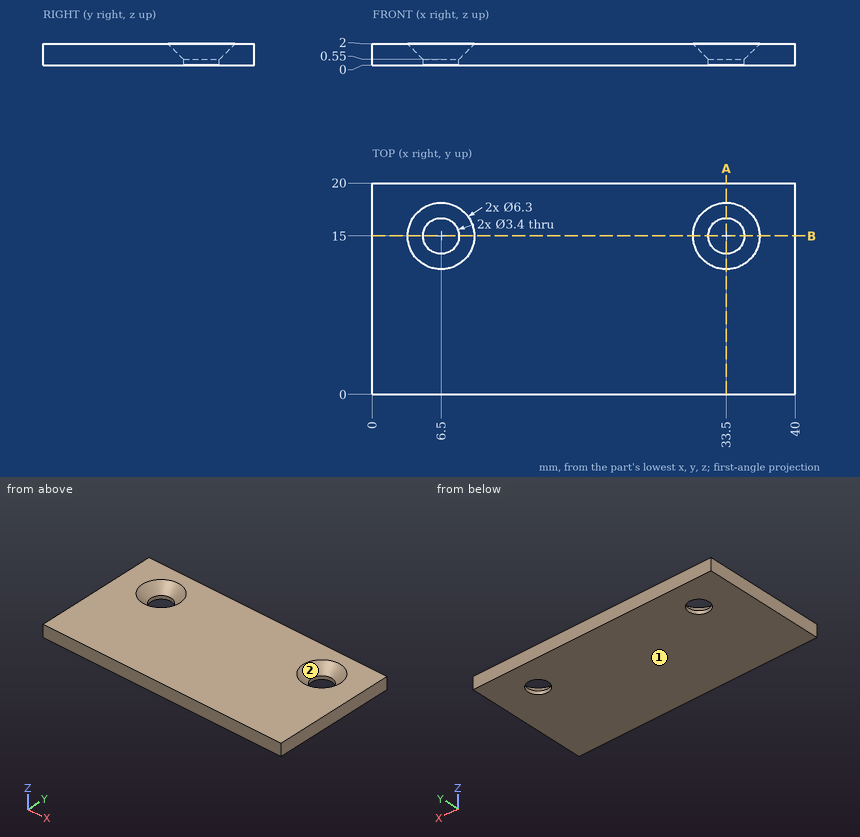
The drawing under review shows one solid part. Ordinate dimensions are in mm from its lowest x, y, z. Coordinates: 2 decimals unless noted, no trailing zeros. Order: outer loops, then holes, each group sorted by start corner. A loop starts at its lowest first (then second) coordinate and runs counter-clockwise, first axis right, second up. Notation, with made-up numbers: M 3,56.5 L 15,56.5 A21 ccw 15,93.5 Z; hole C -38,34 d6. An arc over 180 degrees is marked long. Use a Markdown table: item, result.
(1) Add section A-A (x = 33.5). Give the boundary of the cut face in (y, z).
Worked answers:
| item | result |
|---|---|
| outline | M 0,0 L 13.3,0 L 13.3,0.55 L 11.85,2 L 0,2 Z; M 16.7,0 L 20,0 L 20,2 L 18.15,2 L 16.7,0.55 Z |
(2) Draft analysis for pull direction X (two halves, no side actions). For the marked faces 1 and 2, state which applies: released by +X, released by -X, zero draft, split by the parting line, or undercut.
Worked answers:
| item | result |
|---|---|
| face 1 | zero draft |
| face 2 | undercut |
(3) For P1, Ø4, axis at x = 6.5, y = 15, coming from the +Z side; P2, Ø4.5, axis at x = 33.5, y = 15, coming from the +Z side, all flat-tipped, find the tip position at first contact; note any pin that passes through.
Worked answers:
| item | result |
|---|---|
| P1 | stops at z = 0.85 |
| P2 | stops at z = 1.1 |
(4) Add section B-B (y = 15). Give the boundary of the cut face in (x, z), then the cut area to 3 significant figures.
Worked answers:
| item | result |
|---|---|
| outline | M 0,0 L 4.8,0 L 4.8,0.55 L 3.35,2 L 0,2 Z; M 8.2,0 L 31.8,0 L 31.8,0.55 L 30.35,2 L 9.65,2 L 8.2,0.55 Z; M 35.2,0 L 40,0 L 40,2 L 36.65,2 L 35.2,0.55 Z |
| area | 62.2 mm2 |
(5) Wall thickness on probe 1 along X at (y, z) = (15, 0.3); probe 2 along Y at (x, z) = (6.5, 0.25); probe 3 along X at (y, z) = (17, 1.7): over which ranges is each line inside the solid? List them lowest first.
Worked answers:
| item | result |
|---|---|
| probe 1 | x = 0 to 4.8, 8.2 to 31.8, 35.2 to 40 |
| probe 2 | y = 0 to 13.3, 16.7 to 20 |
| probe 3 | x = 0 to 4.47, 8.53 to 31.47, 35.53 to 40 |
